Can you work these out from the model? Positions are in its coordinate system, mm. Face numbers are marked on the shaded views. A direction names the side the tool comes from. Round coordinates to 2 decimals unless told otherwise and drop trailing zeros. Loops run counter-clockwise (first coordinate to the right, second up) from the corner with the lowest first, then second, coordinate; pieces in that order, holes last.
(1) Which directions (+Z, -Z, +X, -X, +Y, -Y) give clear straight access to the entire face, cutting with the end or side of a thin tool? Please do the marked faces 3 and 4.
(2) I want a section at A-A on y = -19. Write out the boundary of the cut face in (x, z).
(3) I want a section at B-B on x = -0.25. Give the number of separate pieces and of enclosed holes in the cut face, plus the area to 3 significant figures.
(4) Will these pins go through, and if not, where does the flat tip stop? pin 1 Ø1 at (x, z) = (0.5, 26) entering from -Y; pin 2 Ø6 at (y, z) = (-1, 2) entering from +X; pin 3 Ø2 at (x, y) = (0, 10.5) entering from +Z; pin 4 Ø5.5 at (y, z) = (6.44, 19.82) entering from +X (3 decimals).
(5) Thinking about a two-plate mould opening in Z: for the marked faces 1 and 2, which applies, released by +Z, released by -Z, zero draft, split by the parting line, or undercut?
(6) If I drill on line 1 along Z through (x, y) = (4.75, -23); line 2 along Z through (x, y) = (4, -35); line 3 along X through (y, z) = (29, -21), over which ranges is the centre line in solid material (lowest first)?
from build123d import *

# Parameters (mm, degrees)
BASPROSKE_W        = 6.35
BASPROSKE_H        = 53.975
TOOTHCUT_DEPTH     = 77.59584682
TEETHCUTS_COUNT    = 15
TEETHCUTS_ANGLE    = 336
HUBNEABOTSKE_R     = 38.1
HUBNEARBOTH_DEPTH  = 3.1750254
HUBFAR_START       = 3.1750254
HUBFARSKE_R        = 38.1
HUBFAR_DEPTH       = 3.1750254
BORSKE_R           = 6.35
BORE_DEPTH         = 12.7000508
SKETCH1_R          = 6.35
CUT_EXTRUDE1_DEPTH = 78.297193623
SCALE1_SCALE       = 0.75


with BuildPart() as part:
    # BasProSke → Base-Revolve (revolve)
    with BuildSketch(Plane(origin=(0, 0, 0), x_dir=(1, 0, 0), z_dir=(0, 1, 0)), mode=Mode.PRIVATE) as base_revolve_sk:
        with Locations((3.175, 26.9875)):
            Rectangle(BASPROSKE_W, BASPROSKE_H)
    revolve(base_revolve_sk.sketch.rotate(Axis((-10, 0, 0), (1, 0, 0)), 180), axis=Axis((-10, 0, 0), (1, 0, 0)))

    # TooCutSke → ToothCut (cut, through all)
    with BuildSketch(Plane(origin=(0, 0, 0), x_dir=(0, 0, -1), z_dir=(1, 0, 0))):
        with BuildLine():
            ThreePointArc((3.91547882, 39.492605349), (0, 39.68623), (-3.91547882, 39.492605349))
            ThreePointArc((-3.91547882, 39.492605349), (-5.201686692, 46.882953453), (-9.241355572, 53.20376441))
            ThreePointArc((-9.241355572, 53.20376441), (0, 54.0004), (9.241355572, 53.20376441))
            ThreePointArc((9.241355572, 53.20376441), (5.201686692, 46.882953453), (3.91547882, 39.492605349))
        make_face()
    toothcut = extrude(amount=TOOTHCUT_DEPTH, mode=Mode.SUBTRACT)

    # TeethCuts: ToothCut ×15 about axis
    teethcuts_axis = Axis((-10, 0, 0), (1, 0, 0))
    for i in range(1, TEETHCUTS_COUNT):
        add(toothcut.rotate(teethcuts_axis, i * TEETHCUTS_ANGLE / (TEETHCUTS_COUNT - 1)), mode=Mode.SUBTRACT)

    # HubNeaBotSke → HubNearBoth (add)
    with BuildSketch(Plane.ZY):
        with Locations(Location((0, 0, 0), (0, 0, 180))):
            Circle(HUBNEABOTSKE_R)
    extrude(amount=HUBNEARBOTH_DEPTH)

    # HubFarSke → HubFar (add)
    with BuildSketch(Plane(origin=(6.35, 0, 0), x_dir=(0, 0, -1), z_dir=(1, 0, 0)).offset(HUBFAR_START)):
        Circle(HUBFARSKE_R)
    extrude(amount=-HUBFAR_DEPTH)

    # BorSke → Bore (cut, symmetric)
    with BuildSketch(Plane(origin=(0, 0, 0), x_dir=(0, 0, -1), z_dir=(1, 0, 0))):
        with Locations(Location((0, 0, 0), (0, 0, 180))):
            Circle(BORSKE_R)
    extrude(amount=BORE_DEPTH, both=True, mode=Mode.SUBTRACT)

    # Sketch1 → Cut-Extrude1 (cut, through all)
    with BuildSketch(Plane.ZY.offset(3.1750254)):
        with Locations((26.638896337, 8.655502106)):
            Circle(SKETCH1_R)
    extrude(amount=-CUT_EXTRUDE1_DEPTH, mode=Mode.SUBTRACT)


with BuildPart() as part_1:
    # Scale1: scaled about (3.175, -0.202804759, -0.624168867)
    add(part.part.scale(SCALE1_SCALE).moved(Location((0.79375, -0.05070119, -0.156042217))))


solid = part_1.part
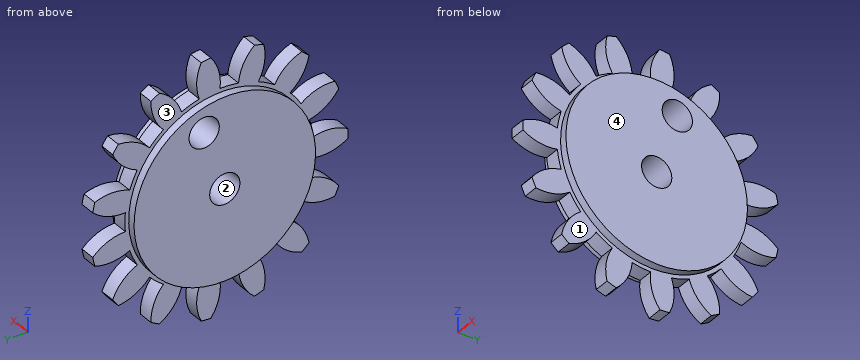
Filled sheet:
1. face 3: -X
1. face 4: +Z, -Z, +X, +Y, -Y
2. outline: (-1.59, -21.54) - (0.79, -21.54) - (0.79, -26.69) - (5.56, -26.69) - (5.56, -21.54) - (7.94, -21.54) - (7.94, 21.23) - (5.56, 21.23) - (5.56, 26.37) - (0.79, 26.37) - (0.79, 21.23) - (-1.59, 21.23) - close
3. separate pieces: 1
3. enclosed holes: 2
3. area: 2,420 mm2
4. pin 1: stops at y = -27.58
4. pin 2: stops at x = 7.94
4. pin 3: stops at z = 27.9
4. pin 4: passes through
5. face 1: zero draft
5. face 2: undercut
6. line 1: z = -30 to -20.47, -19.11 to 18.8, 20.15 to 29.68
6. line 2: z = -18.13 to -12.3, -3.69 to 3.38, 11.99 to 17.82
6. line 3: x = 0.79 to 5.56
